Read the model definition and answer for the solid it produces. Units are mm, in the model's axes. A direction names the side the tool comes from. Coordinates: 2 decimals unless noted, no trailing zeros. Loops run counter-clockwise (first coordinate to the right, second up) from the corner with the lowest first, then second, coordinate; pieces in that order, holes last. Notation, with made-up numbers: (9, 86) -> (64, 86) arc R33 ccw to (64, 124) -> close; hole circle Ø4 at (43, 14.25). An arc over 180 degrees is marked (long way). Answer as a JSON object with one key per item and string values. Group by question number.
1) Section C-C, the plane x = 3.25 is taken. Give the vertices of the cut face in (y, z), plus the area to 3 significant figures.
2) Determine the mould class of faces 1 (the face through (1.617, -0.67, 11.465)), 2 (the face through (-1, 5.6, 4)), 3 (the face through (-3.55, -1, -2)) for opening direction X: released by +X, released by -X, zero draft, split by the parting line, or undercut.
3) Section D-D, the plane x = 1 is taken. Count the separate pieces of the cut face and the enclosed holes in it, plus the area to 3 significant figures.
4) Consider probe 1 along Z at (x, y) = (1, -3.7); probe 2 along X at (y, z) = (-3.75, -3.7); probe 3 along Z at (x, y) = (2.25, 3.5). Determine where each line is inside the solid, lowest interval first. Write a range as [from, to].
5) Section B-B, the plane z = 10.5 is taken. Give the vertices of the cut face in (x, y).
6) Section A-A, the plane x = 0 is taken. Give the vertices of the cut face in (y, z).
7) Which of the six approach directions +Z, -Z, +X, -X, +Y, -Y give full straight-line access (tool end or side, diameter ignored) to faces 4 (the face through (3, 1, 10)), 5 (the face through (-4.05, -1, -2)), 6 (the face through (0, 3, 9.5))?
8) Flat-ended cylindrical pins translate along their axes: P1, Ø2, axis at y = -1.5, z = -2.5, coming from the -X side; P2, Ø2, axis at x = 0.5, y = 3, coming from the -Z side; P3, Ø3, axis at x = 0.5, z = -3, coming from the +Y side. Find the tip coordinate at first contact, or state that the pin passes through.
from build123d import *

# Parameters (mm, degrees)
SKETCH3_W           = 9
SKETCH3_H           = 10.5
SKETCH3_W_2         = 1.5
SKETCH3_H_2         = 0.5
SKETCH3_W_3         = 0.5
SKETCH3_H_3         = 1.5
BOSS_EXTRUDE1_DEPTH = 9
SKETCH5_R           = 2.95
BOSS_EXTRUDE4_DEPTH = 1
SKETCH5_3_R         = 2.95
SKETCH5_3_R_2       = 1.75
BOSS_EXTRUDE5_DEPTH = 5
SKETCH3_3_W         = 1.5
SKETCH3_3_H         = 0.5
SKETCH3_3_W_2       = 0.5
SKETCH3_3_H_2       = 1.5
BOSS_EXTRUDE6_DEPTH = 3.7
SKETCH6_R           = 1.3
SKETCH6_R_2         = 0.6
BOSS_EXTRUDE7_DEPTH = 0.5
CUT_EXTRUDE1_DEPTH  = 3.7
CUT_EXTRUDE2_DEPTH  = 3.7
SKETCH7_3_R         = 1.3
SKETCH7_3_R_2       = 0.6
BOSS_EXTRUDE8_DEPTH = 0.5
CUT_EXTRUDE3_DEPTH  = 3.7
SKETCH8_3_R         = 1.3
SKETCH8_3_R_2       = 0.6
BOSS_EXTRUDE9_DEPTH = 0.5
CHAMFER1_SIZE       = 0.5


with BuildPart() as part:
    # Sketch3 → Boss-Extrude1 (new body)
    with BuildSketch(Plane.XY):
        with Locations((-0.5, 0.35)):
            Rectangle(SKETCH3_W, SKETCH3_H)
        with Locations((1, -3.7)):
            Rectangle(SKETCH3_W_2, SKETCH3_H_2, mode=Mode.SUBTRACT)
        with Locations((-3.8, -1.4)):
            Rectangle(SKETCH3_W_3, SKETCH3_H_3, mode=Mode.SUBTRACT)
        with Locations((1, 4.4)):
            Rectangle(SKETCH3_W_2, SKETCH3_H_2, mode=Mode.SUBTRACT)
        with Locations((1, -3.7)):
            Rectangle(SKETCH3_W_2, SKETCH3_H_2)
        with Locations((-3.8, -1.4)):
            Rectangle(SKETCH3_W_3, SKETCH3_H_3)
        with Locations((1, 4.4)):
            Rectangle(SKETCH3_W_2, SKETCH3_H_2)
    extrude(amount=BOSS_EXTRUDE1_DEPTH)

    # Sketch5 → Boss-Extrude4 (add)
    with BuildSketch(Plane.XY.offset(9)):
        with BuildLine():
            ThreePointArc((-4, 0), (-3.645751311, -1.645751311), (-2.645751311, -3))
            Line((-2.645751311, -3), (2.645751311, -3))
            ThreePointArc((2.645751311, -3), (3.645751311, -1.645751311), (4, 0))
            ThreePointArc((4, 0), (3.645751311, 1.645751311), (2.645751311, 3))
            Line((2.645751311, 3), (-2.645751311, 3))
            ThreePointArc((-2.645751311, 3), (-3.645751311, 1.645751311), (-4, 0))
        make_face()
        Circle(SKETCH5_R, mode=Mode.SUBTRACT)
    extrude(amount=BOSS_EXTRUDE4_DEPTH)

    # Sketch5<3> → Boss-Extrude5 (add)
    with BuildSketch(Plane.XY.offset(9)):
        Circle(SKETCH5_3_R)
        Circle(SKETCH5_3_R_2, mode=Mode.SUBTRACT)
    extrude(amount=BOSS_EXTRUDE5_DEPTH)

    # Sketch3<3> → Boss-Extrude6 (add)
    with BuildSketch(Plane.XY):
        with Locations((1, -3.7)):
            Rectangle(SKETCH3_3_W, SKETCH3_3_H)
        with Locations((-3.8, -1.4)):
            Rectangle(SKETCH3_3_W_2, SKETCH3_3_H_2)
        with Locations((1, 4.4)):
            Rectangle(SKETCH3_3_W, SKETCH3_3_H)
    extrude(amount=-BOSS_EXTRUDE6_DEPTH)

    # Sketch6 → Boss-Extrude7 (add)
    with BuildSketch(Plane.XZ.offset(3.95)):
        with Locations((1, -3.7)):
            Circle(SKETCH6_R)
        with Locations((1, -3.7)):
            Circle(SKETCH6_R_2, mode=Mode.SUBTRACT)
    extrude(amount=-BOSS_EXTRUDE7_DEPTH)

    # Sketch6<2> → Cut-Extrude1 (cut)
    with BuildSketch(Plane.XZ.offset(3.95)):
        with BuildLine():
            Line((0.4, -3.7), (1.6, -3.7))
            ThreePointArc((1.6, -3.7), (1, -3.1), (0.4, -3.7))
        make_face()
        with BuildLine():
            ThreePointArc((0.4, -3.7), (1, -4.3), (1.6, -3.7))
            Line((1.6, -3.7), (0.4, -3.7))
        make_face()
    extrude(amount=-CUT_EXTRUDE1_DEPTH, mode=Mode.SUBTRACT)

    # Sketch7 → Cut-Extrude2 (cut)
    with BuildSketch(Plane.XZ.offset(-4.15)):
        with BuildLine():
            Line((0.4, -3.7), (1.6, -3.7))
            ThreePointArc((1.6, -3.7), (1, -3.1), (0.4, -3.7))
        make_face()
        with BuildLine():
            ThreePointArc((0.4, -3.7), (1, -4.3), (1.6, -3.7))
            Line((1.6, -3.7), (0.4, -3.7))
        make_face()
    extrude(amount=-CUT_EXTRUDE2_DEPTH, mode=Mode.SUBTRACT)

    # Sketch7<3> → Boss-Extrude8 (add)
    with BuildSketch(Plane.XZ.offset(-4.15)):
        with Locations((1, -3.7)):
            Circle(SKETCH7_3_R)
        with Locations(Location((1, -3.7, 0), (0, 0, 270))):
            Circle(SKETCH7_3_R_2, mode=Mode.SUBTRACT)
    extrude(amount=-BOSS_EXTRUDE8_DEPTH)

    # Sketch8 → Cut-Extrude3 (cut)
    with BuildSketch(Plane.ZY.offset(4.05)):
        with BuildLine():
            ThreePointArc((-3.7, -2), (-3.275735931, -1.824264069), (-3.1, -1.4))
            ThreePointArc((-3.1, -1.4), (-3.275735931, -0.975735931), (-3.7, -0.8))
            Line((-3.7, -0.8), (-3.7, -2))
        make_face()
        with BuildLine():
            Line((-3.7, -2), (-3.7, -0.8))
            ThreePointArc((-3.7, -0.8), (-4.3, -1.4), (-3.7, -2))
        make_face()
    extrude(amount=-CUT_EXTRUDE3_DEPTH, mode=Mode.SUBTRACT)

    # Sketch8<3> → Boss-Extrude9 (add)
    with BuildSketch(Plane.ZY.offset(4.05)):
        with Locations((-3.7, -1.4)):
            Circle(SKETCH8_3_R)
        with Locations((-3.7, -1.4)):
            Circle(SKETCH8_3_R_2, mode=Mode.SUBTRACT)
    extrude(amount=-BOSS_EXTRUDE9_DEPTH)

    # Chamfer1
    chamfer1_edges = [part.edges().sort_by_distance(p)[0] for p in [
        (-2.95, 0, 14),
    ]]
    chamfer(chamfer1_edges, length=CHAMFER1_SIZE)


solid = part.part
Determined:
{
 "1": {"outline": "(-4.9, 0) -> (5.6, 0) -> (5.6, 9) -> (2.33, 9) -> (2.33, 10) -> (-2.33, 10) -> (-2.33, 9) -> (-4.9, 9) -> close", "area": "99.2 mm²"},
 "2": {"face 1": "undercut", "face 2": "zero draft", "face 3": "released by +X"},
 "3": {"separate pieces": "3", "enclosed holes": "0", "area": "112 mm²"},
 "4": {"probe 1": "[-5, -4.3], [-3.1, 9]", "probe 2": "[-0.3, 0.4], [1.6, 2.3]", "probe 3": "[0, 9]"},
 "5": {"outline": "circle Ø5.9 at (0, 0); hole circle Ø3.5 at (0, 0)"},
 "6": {"outline": "(-4.9, 0) -> (5.6, 0) -> (5.6, 9) -> (3, 9) -> (3, 10) -> (2.95, 10) -> (2.95, 13.5) -> (2.45, 14) -> (1.75, 14) -> (1.75, 9) -> (-1.75, 9) -> (-1.75, 14) -> (-2.45, 14) -> (-2.95, 13.5) -> (-2.95, 10) -> (-3, 10) -> (-3, 9) -> (-4.9, 9) -> close; (-3.95, -4.53) -> (-3.45, -4.53) -> (-3.45, -2.87) -> (-3.95, -2.87) -> close; (4.15, -4.53) -> (4.65, -4.53) -> (4.65, -2.87) -> (4.15, -2.87) -> close"},
 "7": {"face 4": "+Z", "face 5": "-Z, -X, +Y, -Y", "face 6": "+Z, +X, -X, +Y"},
 "8": {"P1": "x = -4.05", "P2": "z = 0", "P3": "y = 4.65"}
}
